from build123d import *

# Parameters (mm, degrees)
EXTRUSION1_DEPTH = 200
ESQUISSE3_R      = 1.5
EXTRUSION3_DEPTH = 150
ESQUISSE2_R      = 1.5
EXTRUSION4_DEPTH = 100


with BuildPart() as part:
    # Esquisse1 → Extrusion1 (new body)
    with BuildSketch(Plane.XY):
        Polygon((-18.113475854, 1.818947368), (-18.113475854, -18.181052632), (1.886524146, -18.181052632), (1.886524146, -16.681052632), (-16.613475854, -16.681052632), (-16.613475854, 1.818947368), align=None)
    extrude(amount=EXTRUSION1_DEPTH)

    # Esquisse3 → Extrusion3 (cut)
    with BuildSketch(Plane(origin=(-16.613475854, 0, 0), x_dir=(0, 0, -1), z_dir=(1, 0, 0))):
        with Locations((-10, -8.181052632)):
            Circle(ESQUISSE3_R)
        with Locations((-188.5, -8.181052632)):
            Circle(ESQUISSE3_R)
    extrude(amount=-EXTRUSION3_DEPTH, mode=Mode.SUBTRACT)

    # Esquisse2 → Extrusion4 (cut)
    with BuildSketch(Plane(origin=(0, -16.681052632, 0), x_dir=(-1, 0, 0), z_dir=(0, 1, 0))):
        with Locations((8.113475854, 170)):
            Circle(ESQUISSE2_R)
        with Locations((8.113475854, 30)):
            Circle(ESQUISSE2_R)
    extrude(amount=-EXTRUSION4_DEPTH, mode=Mode.SUBTRACT)


solid = part.part
Input: part model. Units: mm. Frame: model coordinates. A direction names the side the tool comes from. Round coordinates to 2 decimals unless told otherwise and drop trailing zeros. Loops run counter-clockwise (first coordinate to the right, second up) from the corner with the lowest first, then second, coordinate; pieces in that order, holes last. Notation, with made-up numbers: (-11.5, -12.75) -> (-5.5, -12.75) arc R18 ccw to (-5.5, 5.25) -> close; hole circle Ø8 at (-21, -17.5). An arc over 180 degrees is marked (long way). Answer as a JSON object with one key per item and string values. Group by question number.
1) Section query A-A on z = 94. Output: boundary loops of the cut face in (x, y).
2) Reachability of faces 1 (the flat face through (-8, -18.181, 99)), 2 (the flat face through (-16.613, -8, 99)) from +Z, -Z, +X, -X, +Y, -Y: full face, straight path, thin tool, end or side. Return the list, or none.
3) Pin query (flat end, axial travel): pin 1 (10 mm diameter, centred on x = -11.5, z = 178.5, fed in from +Y); pin 2 (4 mm diameter, centred on y = -8.18, z = 188.5, fed in from +X); pin 3 (12 mm diameter, centred on x = -7.5, y = -5.5, fed in from -Z). Return the tip coordinate at first contact, or that it passes through.
4) Section query B-B on x = -4.75. Output: boundary loops of the cut face in (y, z).
5) Ray query, L1, parallel to Y at x = -2.25, z = 145.5; L2, parallel to X at y = -7, z = 42. Return the intervals inside material, ascending.
Reply:
{
 "1": {"outline": "(-18.11, -18.18) -> (1.89, -18.18) -> (1.89, -16.68) -> (-16.61, -16.68) -> (-16.61, 1.82) -> (-18.11, 1.82) -> close"},
 "2": {"face 1": "+Z, -Z, +X, -X, -Y", "face 2": "+Z, -Z, +X, +Y"},
 "3": {"pin 1": "stops at y = -16.68", "pin 2": "stops at x = -16.61", "pin 3": "passes through"},
 "4": {"outline": "(-18.18, 0) -> (-16.68, 0) -> (-16.68, 200) -> (-18.18, 200) -> close"},
 "5": {"L1": "y = -18.18 to -16.68", "L2": "x = -18.11 to -16.61"}
}
